Solid Edge part; units mm, degrees
sketch "Sketch1" plane through (0, 0, 0) normal (0, 0, 1) x (1, 0, 0)
  line L0 (-15.3863, -14.0712) -> (15.6137, -14.0712)
  line L1 (15.6137, -14.0712) -> (15.6137, 16.9288)
  line L2 (15.6137, 16.9288) -> (-15.3863, 16.9288)
  line L3 (-15.3863, 16.9288) -> (-15.3863, -14.0712)
extrude "Protrusion1" add sketch "Sketch1" along normal blind 2
sketch "Sketch2" plane through (0.1137, 1.4288, 2) normal (0, 0, 1) x (1, 0, 0)
  line L0 (-18, -18) -> (18, -18)
  line L1 (18, -18) -> (18, 18)
  line L2 (18, 18) -> (-18, 18)
  line L3 (-18, 18) -> (-18, -18)
extrude "ExtrudedProtrusion_3" add sketch "Sketch2" along normal blind 2
sketch "Sketch3" plane through (0.1137, 1.4288, 0) normal (0, 0, -1) x (1, 0, 0)
  line L0 (-13.5, -13.5) -> (13.5, -13.5)
  line L1 (13.5, -13.5) -> (13.5, 13.5)
  line L2 (13.5, 13.5) -> (-13.5, 13.5)
  line L3 (-13.5, 13.5) -> (-13.5, -13.5)
extrude "ExtrudedCutout_1" cut sketch "Sketch3" against normal blind 2
sketch "Sketch4" plane through (0.1137, 1.4288, 4) normal (0, 0, 1) x (-1, 0, 0)
  line L0 (-18, -2.5) -> (-18, 2.5)
  arc A0 (-18, 2.5) -> (-18, -2.5) centre (-18, 0) ccw
  line L1 (18, -2.5) -> (18, 2.5)
  arc A1 (18, 2.5) -> (18, -2.5) centre (18, 0) cw
extrude "ExtrudedProtrusion_4" add sketch "Sketch4" against normal blind 2
The listing builds one solid part. Answer for the finished solid, in the listing's coordinates (mm). A direction names the side the tool comes from. Give positions to 0.01 mm unless a question says otherwise; leave off trailing zeros. Order: outer loops, then holes, each group sorted by start corner. A loop starts at its lowest first (then second) coordinate and runs counter-clockwise, first axis right, second up. Notation, with made-up numbers: (89, 31) - (110, 31) arc R20 ccw to (110, 36) - close; hole circle Ø10 at (15, 35). An arc over 180 degrees is marked (long way). Use one line per item in the form item = value.
1) Find section C-C on x = -4. Determine the outline of the cut face in (y, z), and give its area (3 significant figures).
Verdict:
outline = (-16.57, 2) - (-14.07, 2) - (-14.07, 0) - (-12.07, 0) - (-12.07, 2) - (14.93, 2) - (14.93, 0) - (16.93, 0) - (16.93, 2) - (19.43, 2) - (19.43, 4) - (-16.57, 4) - close
area = 80.0 mm^2
2) For faces 1 (the flat face through (-17.886, 12, 3)), 2 (the flat face through (18.114, 12, 3)), 3 (the flat face through (-13.386, 1, 1)), 4 (the flat face through (0, -14.071, 1)), determine the directions among +Z, -Z, +X, -X, +Y, -Y from which every point of the face is accessible in a straight line to the end or side of a thin tool.
Verdict:
face_1 = +Z, -Z, -X, +Y
face_2 = +Z, -Z, +X, +Y
face_3 = -Z
face_4 = -Z, +X, -X, -Y
3) Each of these flat-tipped pins is pushed along its axis until it touches: pin 1 (2 mm diameter, centred on y = -3, z = 1.5, fed in from -X); pin 2 (0.6 mm diameter, centred on x = -2, z = 0.5, fed in from -Y); pin 3 (2 mm diameter, centred on y = 13, z = 2.5, fed in from +X). Where does it stop, or does it pass through?
Verdict:
pin_1 = -17.89
pin_2 = -14.07
pin_3 = 18.11
4) Find section D-D on z = 3.25. Determine the outline of the cut face in (x, y), and give its area (3 significant figures).
Verdict:
outline = (-17.89, -16.57) - (18.11, -16.57) - (18.11, -1.07) arc R2.5 ccw to (18.11, 3.93) - (18.11, 19.43) - (-17.89, 19.43) - (-17.89, 3.93) arc R2.5 ccw to (-17.89, -1.07) - close
area = 1,320 mm^2
5) Find section A-A on z = 0.8. Determine the outline of the cut face in (x, y).
Verdict:
outline = (-15.39, -14.07) - (15.61, -14.07) - (15.61, 16.93) - (-15.39, 16.93) - close; hole (-13.39, -12.07) - (13.61, -12.07) - (13.61, 14.93) - (-13.39, 14.93) - close
6) The mould has two halves that part along Y. Classify faces 5 (the flat face through (14, 2, 0)), 6 (the flat face through (0, 19.429, 3)), 7 (the flat face through (0, 2, 2)): released by +Y, released by -Y, zero draft, split by the parting line, or undercut.
Verdict:
face_5 = zero draft
face_6 = released by +Y
face_7 = undercut
7) Find section B-B on y = -13. Determine the outline of the cut face in (x, z).
Verdict:
outline = (-17.89, 2) - (-15.39, 2) - (-15.39, 0) - (15.61, 0) - (15.61, 2) - (18.11, 2) - (18.11, 4) - (-17.89, 4) - close
8) Consider probe 1 along X at (y, z) = (13, 0.8); probe 2 along Y at (x, z) = (1, 0.9); probe 3 along X at (y, z) = (-4.5, 3.4). Determine where each line is inside the solid, lowest interval first. Write a range as [from, to].
Verdict:
probe_1 = [-15.39, -13.39], [13.61, 15.61]
probe_2 = [-14.07, -12.07], [14.93, 16.93]
probe_3 = [-17.89, 18.11]
